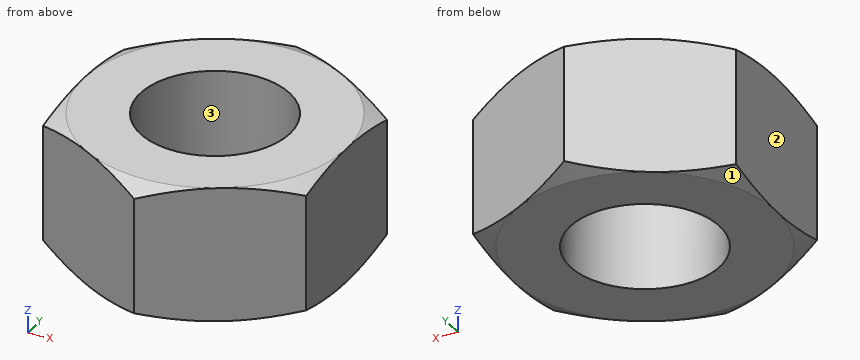
from build123d import *

# Parameters (mm, degrees)
F0_R     = 3.175
F1_DEPTH = 2.8702


with BuildPart() as f1:
    # F0 (on Top) → F1 (new body, symmetric)
    with BuildSketch(Plane.XY):
        Polygon((0, -6.423137), (5.5626, -3.211569), (5.5626, 3.211569), (0, 6.423137), (-5.5626, 3.211569), (-5.5626, -3.211569), align=None)
        Circle(F0_R, mode=Mode.SUBTRACT)
    extrude(amount=F1_DEPTH, both=True)

    # F2 (on Front) → F3 (revolve, cut)
    with BuildSketch(Plane.XZ):
        Polygon((6.773051, 2.8702), (5.5626, 2.8702), (6.773051, 2.301839), align=None)
    revolve(axis=Axis((0, 0, 2.8702), (0, 0, 1)), mode=Mode.SUBTRACT)

    # F2 (on Front) → F4 (revolve, cut)
    with BuildSketch(Plane.XZ):
        Polygon((6.773051, -2.8702), (6.773051, -2.301839), (5.5626, -2.8702), align=None)
    revolve(axis=Axis((0, 0, -2.8702), (0, 0, 1)), mode=Mode.SUBTRACT)


solid = f1.part
Part model, mm, in its own coordinate system. Face numbers are marked on the shaded views. Coordinates: 2 decimals unless noted, no trailing zeros. Loops run counter-clockwise (first coordinate to the right, second up) from the corner with the lowest first, then second, coordinate; pieces in that order, holes last. Notation, with made-up numbers: M 28.5,-22.75 L 72.5,-22.75 A7 ccw 72.5,-11.75 Z; hole C 52,49 d8. An arc over 180 degrees is marked long. Use a Markdown table: item, result. Add a question column.
Q1. Probe L1, parallel to X at y = -2, z = 0.65; L2, parallel to Y at x = 2.5, z = 0.7; L3, parallel to Y at x = 1, z = -1.3. List the from-to ranges inside material, lowest first.
Q2. Mould opens along Y. For the marked faces 1, 2 and 3 say: +Y half, -Y half, draft (parallel to the pull), parting line (faces both ways), or undercut.
Q3. Pin check, flat tips, straight feed: P1, Ø2, axis at x = -1.5, z = 0.5, coming from the -Y side; P2, Ø1.5, axis at x = -3.5, z = 0, coming from the -Y side; P3, Ø5, axis at x = 0, y = 0, coming from the +Z side. Stop position of each tip, or through.
Q4. Cut at A-A (z = -0.9). Write the cut outline in (x, y) (3 decimals), and give its area (3 significant figures).
Worked out:
| question | item | result |
|---|---|---|
| 1 | L1 | x = -5.56 to -2.47, 2.47 to 5.56 |
| 1 | L2 | y = -4.98 to -1.96, 1.96 to 4.98 |
| 1 | L3 | y = -5.85 to -3.01, 3.01 to 5.85 |
| 2 | face 1 | +Y half |
| 2 | face 2 | draft |
| 2 | face 3 | undercut |
| 3 | P1 | stops at y = -6.13 |
| 3 | P2 | stops at y = -4.84 |
| 3 | P3 | passes through |
| 4 | outline | M -5.563,-3.212 L 0,-6.423 L 5.563,-3.212 L 5.563,3.212 L 0,6.423 L -5.563,3.212 Z; hole C 0,0 d6.35 |
| 4 | area | 75.5 mm2 |
